from build123d import *

# Parameters (mm, degrees)
F0_W     = 3.175
F0_H     = 635
F0_W_2   = 327.025
F0_W_3   = 203.2
F0_H_2   = 508
F0_W_4   = 330.2
F0_H_3   = 147.32
F1_DEPTH = 323.85
F2_DEPTH = 6.35
F3_DEPTH = 76.2
F4_W     = 196.85
F4_H     = 660.4
F5_DEPTH = 19.05
F6_DEPTH = 12.7


with BuildPart() as f1:
    # F0 (on Front) → F1 (new body)
    with BuildSketch(Plane.XZ):
        Polygon((0, -101.6), (0, 0), (-3.175, 0), (-330.2, 0), (-330.2, -101.6), align=None)
        with Locations((-1.5875, 317.5)):
            Rectangle(F0_W, F0_H)
        Polygon((3.175, 0), (0, 0), (0, -101.6), (330.2, -101.6), (330.2, 0), align=None)
        with Locations((1.5875, 317.5)):
            Rectangle(F0_W, F0_H)
        with Locations((-166.6875, 317.5)):
            Rectangle(F0_W_2, F0_H)
        with Locations((-165.1, 317.5)):
            Rectangle(F0_W_3, F0_H_2, mode=Mode.SUBTRACT)
        Polygon((-3.175, 635), (0, 635), (0, 640.08), (-330.2, 640.08), (-330.2, 635), align=None)
        Polygon((0, 640.08), (0, 635), (3.175, 635), (330.2, 635), (330.2, 640.08), align=None)
        with Locations((166.6875, 317.5)):
            Rectangle(F0_W_2, F0_H)
        with Locations((165.1, 317.5)):
            Rectangle(F0_W_3, F0_H_2, mode=Mode.SUBTRACT)
        with Locations((-165.1, 713.74)):
            Rectangle(F0_W_4, F0_H_3)
        with Locations((165.1, 713.74)):
            Rectangle(F0_W_4, F0_H_3)
        with Locations((-165.1, 317.5)):
            Rectangle(F0_W_3, F0_H_2)
        with Locations((165.1, 317.5)):
            Rectangle(F0_W_3, F0_H_2)
    extrude(amount=-F1_DEPTH)

    # F0 (on Front) → F2 (cut)
    with BuildSketch(Plane.XZ):
        Polygon((0, -101.6), (0, 0), (-3.175, 0), (-330.2, 0), (-330.2, -101.6), align=None)
        with Locations((-1.5875, 317.5)):
            Rectangle(F0_W, F0_H)
        with Locations((1.5875, 317.5)):
            Rectangle(F0_W, F0_H)
        Polygon((-3.175, 635), (0, 635), (0, 640.08), (-330.2, 640.08), (-330.2, 635), align=None)
        Polygon((0, 640.08), (0, 635), (3.175, 635), (330.2, 635), (330.2, 640.08), align=None)
        with Locations((-165.1, 317.5)):
            Rectangle(F0_W_3, F0_H_2)
        with Locations((165.1, 317.5)):
            Rectangle(F0_W_3, F0_H_2)
    extrude(amount=-F2_DEPTH, mode=Mode.SUBTRACT)

    # F0 (on Front) → F3 (cut)
    with BuildSketch(Plane.XZ):
        Polygon((0, -101.6), (0, 0), (-3.175, 0), (-330.2, 0), (-330.2, -101.6), align=None)
        Polygon((3.175, 0), (0, 0), (0, -101.6), (330.2, -101.6), (330.2, 0), align=None)
    extrude(amount=-F3_DEPTH, mode=Mode.SUBTRACT)

    # F4 (on face) → F5 (join)
    with BuildSketch(Plane(origin=(-330.2, 0, 0), x_dir=(0, -1, 0), z_dir=(-1, 0, 0))):
        Polygon((0, 787.4), (-323.85, 787.4), (-323.85, 0), (-76.2, 0), (0, 0), (0, 635), (-6.35, 635), (-6.35, 640.08), (0, 640.08), align=None)
        with Locations((-161.925, 393.7)):
            Rectangle(F4_W, F4_H, mode=Mode.SUBTRACT)
    extrude(amount=F5_DEPTH)

    # F6 (add): a face of the model
    f6_faces = [f1.faces().sort_by_distance(p)[0] for p in [
        (-330.2, 161.925, 393.7),
    ]]
    extrude(f6_faces, amount=F6_DEPTH)


solid = f1.part
Here's how the part is built. I have some questions about the finished solid (model axes, mm). A direction names the side the tool comes from. Round coordinates to 2 decimals unless told otherwise and drop trailing zeros. Write each loop counter-clockwise with the first axis right and the second up, starting at its lowest first coordinate (ties: lowest second). Pieces come first, ordered by that corner, then holes. Notation, with made-up numbers: (46.5, 23) -> (52.5, 23) arc R22 cw to (52.5, 50) -> close; hole circle Ø2 at (-35.75, 52). An arc over 180 degrees is marked (long way). One line per item, written item: value.
1) We'd pull the mould along Z, two halves only. Please class faces 6 (the face through (-58, 0, 313)), 7 (the face through (-167, 6.35, 321)), 8 (the face through (-5, 160, 787.4)), 9 (the face through (-5, 198, -101.6)): released by +Z, released by -Z, zero draft, split by the parting line, or undercut.
Filled sheet:
face 6: zero draft
face 7: undercut
face 8: released by +Z
face 9: released by -Z
2) Suppose I cut it at C-C on y = 44. List the corners of the cut face in (x, z) for me, plus the area to 3 significant figures.
Filled sheet:
outline: (-349.25, 0) -> (330.2, 0) -> (330.2, 787.4) -> (-349.25, 787.4) -> close
area: 535,000 mm2
3) I'm going to push a flat-ended pin straight in: pin 1 Ø5 at (x, y) = (7, 4) entering from -Z. Where does the tip first touch, or does it pass through?
Filled sheet:
pin 1: stops at z = 0
4) For faces 1 (the face through (-5, 76.2, -50)), 2 (the face through (-330.2, 198, -50)), 3 (the face through (-349.25, 272, 399)), 4 (the face through (-342.9, 161, 398)), 5 (the face through (164, 6.35, 321)), which set-ups out of +Z, -Z, +X, -X, +Y, -Y let a thin tool reach every point of the face, with its end or its side?
Filled sheet:
face 1: -Z, +X, -X, -Y
face 2: -Z, -X, +Y, -Y
face 3: +Z, -Z, -X, +Y, -Y
face 4: -X
face 5: -Y
5) Suppose I cut it at B-B on x = 160.5. List the corners of the cut face in (y, z) for me.
Filled sheet:
outline: (0, 0) -> (76.2, 0) -> (76.2, -101.6) -> (323.85, -101.6) -> (323.85, 787.4) -> (0, 787.4) -> (0, 640.08) -> (6.35, 640.08) -> (6.35, 635) -> (0, 635) -> (0, 571.5) -> (6.35, 571.5) -> (6.35, 63.5) -> (0, 63.5) -> close
6) Suppose I cut it at A-A on z = 163.5. List the corners of the cut face in (x, y) for me (3 decimals).
Filled sheet:
outline: (-349.25, 0) -> (-266.7, 0) -> (-266.7, 6.35) -> (-63.5, 6.35) -> (-63.5, 0) -> (-3.175, 0) -> (-3.175, 6.35) -> (3.175, 6.35) -> (3.175, 0) -> (63.5, 0) -> (63.5, 6.35) -> (266.7, 6.35) -> (266.7, 0) -> (330.2, 0) -> (330.2, 323.85) -> (-349.25, 323.85) -> (-349.25, 260.35) -> (-342.9, 260.35) -> (-342.9, 63.5) -> (-349.25, 63.5) -> close
7) Suppose I cut it at D-D on x = -293. List the corners of the cut face in (y, z) for me.
Filled sheet:
outline: (0, 0) -> (76.2, 0) -> (76.2, -101.6) -> (323.85, -101.6) -> (323.85, 787.4) -> (0, 787.4) -> (0, 640.08) -> (6.35, 640.08) -> (6.35, 635) -> (0, 635) -> close
8) If I drill on line 1 (X direction, y = 87.5, z = 723.5); line 2 (Y direction, x = 69, z = 389); line 3 (X direction, y = 220.5, z = -17.5), over which ranges is the centre line in solid material (lowest first)? Write a range as [from, to].
Filled sheet:
line 1: x = [-342.9, 330.2]
line 2: y = [6.35, 323.85]
line 3: x = [-330.2, 330.2]
